```python
from build123d import *

# Parameters (mm, degrees)
F1_DEPTH       = 9.5
F3_D           = 8.8
F3_CSINK_D     = 9
F3_CSINK_ANGLE = 90


with BuildPart() as f1:
    # F0 (on Front) → F1 (new body)
    with BuildSketch(Plane.XZ):
        with BuildLine():
            Line((52.5, -38), (75, -38))
            Line((75, -38), (75, 38))
            Line((75, 38), (-75, 38))
            Line((-75, 38), (-75, -38))
            Line((-75, -38), (27.5, -38))
            ThreePointArc((27.5, -38), (40, -26.8485699552), (52.5, -38))
        make_face()
    extrude(amount=F1_DEPTH)

    # F3 (through all)
    with Locations(Plane(origin=(0, 0, 0), x_dir=(1, 0, 0), z_dir=(0, 1, 0))):
        with Locations((-60, -28), (65, -28), (9, 31), (-60, 31), (65, 31), (9, -28)):
            CounterSinkHole(F3_D / 2, F3_CSINK_D / 2, counter_sink_angle=F3_CSINK_ANGLE)


solid = f1.part
```
The listing builds one solid part. Answer for the finished solid, in the listing's coordinates (mm). Give positions to 0.01 mm unless a question says otherwise; leave off trailing zeros. Loops run counter-clockwise (first coordinate to the right, second up) from the corner with the lowest first, then second, coordinate; pieces in that order, holes last. Notation, with made-up numbers: M 18,-30 L 49,-30 A20 cw 49,-10 Z; hole C -29.5,-12.5 d1. An arc over 180 degrees is marked long. One line per item, written item: value.
Q1. A flat-ended cylindrical pin translates along its axis: P1, Ø5.5, axis at x = -60, z = 28, coming from the +Y side. Find the tip coordinate at first contact, or state that the pin passes through.
Working result:
P1: passes through
Q2. A cutting plane is placed at A-A on x = 9. Determine the outline of the cut face in (y, z), then the cut area to 3 significant figures.
Working result:
outline: M -9.5,-38 L 0,-38 L 0,-35.5 L -0.1,-35.4 L -9.5,-35.4 Z; M -9.5,-26.6 L -0.1,-26.6 L 0,-26.5 L 0,23.5 L -0.1,23.6 L -9.5,23.6 Z; M -9.5,32.4 L -0.1,32.4 L 0,32.5 L 0,38 L -9.5,38 Z
area: 555 mm^2
Q3. A cutting plane is placed at B-B on y = -4. Determine the outline of the cut face in (x, z), then the cut area to 3 significant figures.
Working result:
outline: M -75,-38 L 27.5,-38 A12.58 cw 52.5,-38 L 75,-38 L 75,38 L -75,38 Z; hole C -60,-31 d8.8; hole C -60,28 d8.8; hole C 9,-31 d8.8; hole C 9,28 d8.8; hole C 65,-31 d8.8; hole C 65,28 d8.8
area: 10,800 mm^2
Q4. A cutting plane is placed at C-C on z = 28. Determine the outline of the cut face in (x, y).
Working result:
outline: M -75,-9.5 L -64.4,-9.5 L -64.4,-0.1 L -64.5,0 L -75,0 Z; M -55.6,-9.5 L 4.6,-9.5 L 4.6,-0.1 L 4.5,0 L -55.5,0 L -55.6,-0.1 Z; M 13.4,-9.5 L 60.6,-9.5 L 60.6,-0.1 L 60.5,0 L 13.5,0 L 13.4,-0.1 Z; M 69.4,-9.5 L 75,-9.5 L 75,0 L 69.5,0 L 69.4,-0.1 Z
Q5. A cutting plane is placed at D-D on z = -31. Determine the outline of the cut face in (x, y).
Working result:
outline: M -75,-9.5 L -64.4,-9.5 L -64.4,-0.1 L -64.5,0 L -75,0 Z; M -55.6,-9.5 L 4.6,-9.5 L 4.6,-0.1 L 4.5,0 L -55.5,0 L -55.6,-0.1 Z; M 13.4,-9.5 L 30.66,-9.5 L 30.66,0 L 13.5,0 L 13.4,-0.1 Z; M 49.34,-9.5 L 60.6,-9.5 L 60.6,-0.1 L 60.5,0 L 49.34,0 Z; M 69.4,-9.5 L 75,-9.5 L 75,0 L 69.5,0 L 69.4,-0.1 Z
Q6. Determine the mould class of faces 1 (the face through (-1, -9.5, 1)), 2 (the face through (39.74, -4.68, -26.85)), 3 (the face through (4.803, -4.866, 26.678)) for opening direction Z: +Z half, -Z half, draft (parallel to the pull), parting line (faces both ways), or undercut.
Working result:
face 1: draft
face 2: -Z half
face 3: undercut
Q7. Find the intervals of material crossed by line 1 (Z direction, x = 64.5, y = -2.25); line 2 (X direction, y = -5.25, z = 28); line 3 (X direction, y = -2.5, z = -31.5), in increasing order. Write a range as from..to.
Working result:
line 1: z = -38..-35.37, -26.63..23.63, 32.37..38
line 2: x = -75..-64.4, -55.6..4.6, 13.4..60.6, 69.4..75
line 3: x = -75..-64.37, -55.63..4.63, 13.37..30.23, 49.77..60.63, 69.37..75
